Autodesk Inventor part; units mm, degrees
ref_plane "YZ Plane" through (0, 0, 0) normal (1, 0, 0) x (0, 1, 0)
ref_plane "XZ Plane" through (0, 0, 0) normal (0, 1, 0) x (-1, 0, 0)
ref_plane "XY Plane" through (0, 0, 0) normal (0, 0, 1) x (1, 0, 0)
sketch "Sketch1" plane through (0, 0, 0) normal (0, 1, 0) x (-1, 0, 0)
  line L0 (0, 0) -> (130, 0)
  line L1 (130, 0) -> (130, -106)
  line L2 (130, -106) -> (0, -106)
  line L3 (0, -106) -> (0, 0)
  line L4 (130, 0) -> (130, -3)
  line L5 (127, -4.0545) -> (0, -4.0545)
  line L6 (0, -4.0545) -> (3, -4.0545)
  line L7 (3, -4.0545) -> (3, -106)
  line L8 (3, -106) -> (3, -103)
  line L9 (3, -103) -> (3, -101.9174)
  line L10 (3, -103) -> (130, -103)
  line L11 (130, -3) -> (127, -4.0545)
  line L12 (130, -103) -> (127, -103)
  line L13 (127, -103) -> (127, -4.0545)
  line L14 (127, -4.0545) -> (0, -4.0545)
  line L15 (0, 0) -> (0, -106)
  line L16 (0, -106) -> (130, -106)
  line L17 (130, -106) -> (130, 0)
  line L18 (127, -4.0545) -> (127, -103)
  line L19 (127, -103) -> (3, -103)
  line L20 (3, -103) -> (3, -4.0545)
  line L21 (3, -4.0545) -> (127, -4.0545)
  dimension "d0" = 130
  dimension "d1" = 106
  dimension "d2" = 3
  dimension "d3" = 3
  dimension "d4" = 3
  dimension "d5" = 3
sketch "Sketch2" plane through (0, 0, 0) normal (0, 1, 0) x (-1, 0, 0)
  point P0 (0, 0)
extrude "Extrusion1" add sketch "Sketch1" along normal blind 13 contours L0 L1 L11 L5 L3 | L5 L7 L2 L3 | L1 L10 L13 L11 | L1 L2 L7 L10
sketch "Sketch6" plane through (-130, 0, 0) normal (0, 0, 1) x (1, 0, 0)
  line L0 (0, 13) -> (130, 13)
  line L1 (0, 13) -> (130, 13)
  line L2 (130, 13) -> (130, 0)
  line L3 (130, 0) -> (0, 0)
  line L4 (0, 0) -> (0, 13)
extrude "Extrusion3" add sketch "Sketch6" along normal blind 2
sketch "Sketch7" plane through (0, 0, 0) normal (0, -1, 0) x (1, 0, 0)
  line L0 (-130, -106) -> (-130, 2)
  line L1 (-130, 0) -> (0, 0)
  line L2 (0, -106) -> (0, 2)
  line L3 (0, 0) -> (0, 2)
  line L4 (0, 2) -> (-130, 2)
  line L5 (-130, 2) -> (-130, 0)
  point P0 (-130, 2)
extrude "Extrusion4" add sketch "Sketch7" along normal blind 4
sketch "Sketch8" plane through (-130, 0, -106) normal (-1, 0, 0) x (0, 0, 1)
  line L0 (108, 13) -> (108, -4)
  line L1 (0, 0) -> (106, 0)
  line L2 (108, 13) -> (0, 13)
  line L3 (0, 13) -> (0, 0)
  line L4 (0, 0) -> (108, 0)
  line L5 (108, 0) -> (108, 13)
extrude "Extrusion5" add sketch "Sketch8" along normal blind 2
sketch "Sketch9" plane through (0, 0, 0) normal (0, -1, 0) x (1, 0, 0)
  line L0 (0, -106) -> (-132, -106)
  line L1 (-132, -106) -> (-130, -106)
  line L2 (-130, -106) -> (-130, 2.3053)
  line L3 (-127, -4.0545) -> (-127, -103)
  line L4 (-130, 2.3053) -> (-132, 2.3053)
  line L5 (-132, -106) -> (-132, 2)
  line L6 (-132, 2.3053) -> (-132, -106)
  point P0 (0, 0)
  dimension "d20" = 2
extrude "Extrusion6" add sketch "Sketch9" along normal blind 4
sketch "Sketch10" plane through (-132, 0, -106) normal (-1, 0, 0) x (0, 0, 1)
  line L0 (108, 13) -> (108, -4)
  line L1 (108, 0) -> (108, -4)
  line L2 (108, -4) -> (108.3053, -4)
  line L3 (108.3053, 0) -> (108.3053, -4)
  line L4 (108.3053, -4) -> (108.3053, 0)
  line L5 (108, 0) -> (108.3053, 0)
  line L6 (108.3053, 0) -> (108.3053, -4)
  line L7 (108.3053, -4) -> (108, -4)
  point P0 (106, 0)
extrude "Extrusion7" cut sketch "Sketch10" against normal blind 4
sketch "Sketch11" plane through (0, 0, -106) normal (0, 0, -1) x (-1, 0, 0)
  line L0 (0, 13) -> (132, 13)
  line L1 (132, 13) -> (0, 13)
  line L2 (0, 13) -> (0, 0)
  line L3 (0, 0) -> (132, 0)
  line L4 (132, 0) -> (132, 13)
extrude "Extrusion8" add sketch "Sketch11" along normal blind 2
sketch "Sketch12" plane through (0, 0, 0) normal (0, -1, 0) x (1, 0, 0)
  line L0 (-132, 2) -> (-132, -106)
  line L1 (0, -108) -> (-132, -108)
  line L2 (-132, -106) -> (0, -106)
  line L3 (0, -106) -> (0, -108)
  line L4 (0, -108) -> (-132, -108)
  line L5 (-132, -108) -> (-132, -106)
  point P0 (0, 0)
extrude "Extrusion9" add sketch "Sketch12" along normal blind 4
sketch "Sketch13" plane through (0, -4, 2) normal (1, 0, 0) x (0, 0, -1)
  line L0 (0, 17) -> (0, 0)
  line L1 (110.1979, 4) -> (0, 4)
  line L2 (0, 4) -> (0, 17)
  line L3 (0, 17) -> (110.1979, 17)
  line L4 (110.1979, 17) -> (110.1979, 4)
  point P0 (2, 4)
  point P1 (0, 4)
extrude "Extrusion10" add sketch "Sketch13" along normal blind 2
sketch "Sketch14" plane through (0, 0, 0) normal (0, -1, 0) x (1, 0, 0)
  line L0 (-132, -108) -> (0, -108)
  line L1 (2, 2) -> (2, -108.1979)
  line L2 (0, -108) -> (2, -108)
  line L3 (2, -108) -> (2, 2)
  line L4 (2, 2) -> (0, 2)
  line L5 (0, 2) -> (0, -108)
  point P0 (0, 0)
extrude "Extrusion11" add sketch "Sketch14" along normal blind 4
sketch "Sketch15" plane through (0, 0, 0) normal (0, -1, 0) x (1, 0, 0)
  line L0 (2, -108) -> (2, -108.1979)
  line L1 (2, -108.1979) -> (0, -108.1979)
  line L2 (0, -108.1979) -> (0, -108)
  line L3 (0, -108) -> (2, -108)
  line L4 (2, -108) -> (2, -108.1979)
  point P0 (0, 0)
extrude "Extrusion12" cut sketch "Sketch15" against normal blind 15
sketch "Sketch16" plane through (0, 0, -108) normal (0, 0, -1) x (-1, 0, 0)
  point P0 (0, 0)
sketch "Sketch17" plane through (0, -4, 0) normal (0, -1, 0) x (1, 0, 0)
  line L0 (2, 2) -> (-132, 2)
  line L1 (-132, 2) -> (-132, -108)
  line L2 (-132, -108) -> (2, -108)
  line L3 (2, -108) -> (2, 2)
  line L4 (0, -106) -> (-130, -106)
  line L5 (-130, 0) -> (-130, -106)
  line L6 (-130, -106) -> (-130, 0)
  line L7 (-130, 0) -> (0, 0)
  line L8 (0, 0) -> (0, -106)
  line L9 (0, -106) -> (-130, -106)
extrude "Extrusion13" add sketch "Sketch17" along normal blind 2
properties part number "che"
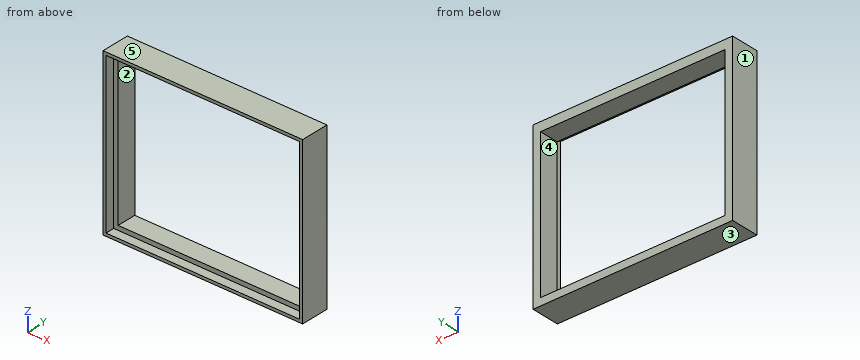
Work out the finished part from the listing and answer in its coordinate system (mm). Face numbers are marked on the shaded views. A direction names the side the tool comes from. Give positions to 0.01 mm unless a question says otherwise; leave off trailing zeros. Order: outer loops, then holes, each group sorted by start corner. A loop starts at its lowest first (then second) coordinate and runs counter-clockwise, first axis right, second up. Notation, with made-up numbers: M 49.5,-38.5 L 82.5,-38.5 A27 ccw 82.5,-15.5 Z; hole C 81.5,32 d4. An arc over 180 degrees is marked long. Return JSON: item names as keys, results as strings.
1) Section A-A, the plane z = -45.5 is taken. Write down the section's boundary in (x, y).
Resolved:
{"outline": "M -132,-6 L -130,-6 L -130,0 L -127,0 L -127,13 L -132,13 Z; M -3,0 L 0,0 L 0,-6 L 2,-6 L 2,13 L -3,13 Z"}
2) Straight lines are drawn through the part: line 1 along Z through (x, y) = (-101, -0.5); line 2 along X through (y, z) = (-0.25, -40); line 3 along Z through (x, y) = (-16.5, 1). For each, find the intervals that lie inside material, in ascending order. Write a range as [from, to].
Resolved:
{"line 1": "[-108, -106], [0, 2]", "line 2": "[-132, -130], [0, 2]", "line 3": "[-108, -103], [-4.05, 2]"}
3) Section D-D, the plane y = -3.25 is taken. Write down the section's boundary in (x, z), plus the area to 3 significant figures.
Resolved:
{"outline": "M -132,-108 L 2,-108 L 2,2 L -132,2 Z; hole M -130,-106 L 0,-106 L 0,0 L -130,0 Z", "area": "960 mm^2"}
4) Section B-B, the plane x = -37 is taken. Write down the section's boundary in (y, z), plus the area to 3 significant figures.
Resolved:
{"outline": "M -6,-108 L 13,-108 L 13,-103 L 0,-103 L 0,-106 L -6,-106 Z; M -6,0 L 0,0 L 0,-4.05 L 13,-4.05 L 13,2 L -6,2 Z", "area": "168 mm^2"}
5) A tool of negligible diameter and unlimited length cuts with its end or side. For the marked faces 1 and 2, from which of +Z, -Z, +X, -X, +Y, -Y can it reach the whole face along a straight path? Write none if from no direction.
Resolved:
{"face 1": "+Z, -Z, -X, +Y, -Y", "face 2": "+Y, -Y"}
6) For a pull along Z with two mould halves and no side action, classify the marked faces 3, 4 and 5 as +Z half, -Z half, draft (parallel to the pull), parting line (faces both ways), or undercut.
Resolved:
{"face 3": "-Z half", "face 4": "undercut", "face 5": "+Z half"}
7) Section C-C, the plane y = 5.5 is taken. Write down the section's boundary in (x, z).
Resolved:
{"outline": "M -132,-108 L 2,-108 L 2,2 L -132,2 Z; hole M -127,-103 L -3,-103 L -3,-4.05 L -127,-4.05 Z"}
